```python
from build123d import *

# Parameters (mm, degrees)
SKETCH1_W           = 80
SKETCH1_H           = 65
BOSS_EXTRUDE1_DEPTH = 3
CUT_EXTRUDE1_DEPTH  = 10
CUT_EXTRUDE2_DEPTH  = 10
SKETCH4_R           = 1.5
CUT_EXTRUDE3_DEPTH  = 10
FILLET1_R           = 3
CUT_EXTRUDE4_DEPTH  = 10


with BuildPart() as part:
    # Sketch1 → Boss-Extrude1 (new body)
    with BuildSketch(Plane(origin=(0, 0, 0), x_dir=(1, 0, 0), z_dir=(0, 1, 0))):
        Rectangle(SKETCH1_W, SKETCH1_H)
    extrude(amount=BOSS_EXTRUDE1_DEPTH)

    # Sketch2 → Cut-Extrude1 (cut)
    with BuildSketch(Plane(origin=(0, 0, 0), x_dir=(-1, 0, 0), z_dir=(0, -1, 0))):
        Polygon((22, 32.5), (22, 14.5), (-1, 14.5), (-1, 26.5), (-18, 26.5), (-18, 14.5), (-40, 14.5), (-40, 32.5), align=None)
        Polygon((-1, -26.5), (-18, -26.5), (-18, -14.5), (-40, -14.5), (-40, -32.5), (22, -32.5), (22, -14.5), (-1, -14.5), align=None)
    extrude(amount=-CUT_EXTRUDE1_DEPTH, mode=Mode.SUBTRACT)

    # Sketch3 → Cut-Extrude2 (cut)
    with BuildSketch(Plane(origin=(0, 3, 0), x_dir=(1, 0, 0), z_dir=(0, 1, 0))):
        Polygon((27, -8.3), (9, -8.3), (9, -5.3), (34, -5.3), (34, -10.3), (27, -10.3), align=None)
        Polygon((34, 5.3), (34, 10.3), (27, 10.3), (27, 8.3), (9, 8.3), (9, 5.3), align=None)
    extrude(amount=-CUT_EXTRUDE2_DEPTH, mode=Mode.SUBTRACT)

    # Sketch4 → Cut-Extrude3 (cut)
    with BuildSketch(Plane(origin=(0, 3, 0), x_dir=(1, 0, 0), z_dir=(0, 1, 0))):
        with Locations(Location((-4, 7, 0), (0, 0, 270))):
            Circle(SKETCH4_R)
        with Locations(Location((13.25, 17.9, 0), (0, 0, 270))):
            Circle(SKETCH4_R)
        with Locations(Location((5.75, 17.9, 0), (0, 0, 270))):
            Circle(SKETCH4_R)
        with Locations(Location((37, 7, 0), (0, 0, 270))):
            Circle(SKETCH4_R)
        with Locations(Location((37, 12, 0), (0, 0, 270))):
            Circle(SKETCH4_R)
        with Locations(Location((-19, 12, 0), (0, 0, 270))):
            Circle(SKETCH4_R)
        with Locations(Location((-27.636753237, 17.892684015, 0), (0, 0, 270))):
            Circle(SKETCH4_R)
        with Locations(Location((-34.28355698, 11.245880272, 0), (0, 0, 270))):
            Circle(SKETCH4_R)
        with Locations(Location((-34.28355698, -11.245880272, 0), (0, 0, 270))):
            Circle(SKETCH4_R)
        with Locations(Location((-27.636753237, -17.892684015, 0), (0, 0, 270))):
            Circle(SKETCH4_R)
        with Locations(Location((-19, -12, 0), (0, 0, 270))):
            Circle(SKETCH4_R)
        with Locations(Location((-4, -7, 0), (0, 0, 270))):
            Circle(SKETCH4_R)
        with Locations(Location((5.75, -17.9, 0), (0, 0, 270))):
            Circle(SKETCH4_R)
        with Locations(Location((13.25, -17.9, 0), (0, 0, 270))):
            Circle(SKETCH4_R)
        with Locations(Location((37, -7, 0), (0, 0, 270))):
            Circle(SKETCH4_R)
        with Locations(Location((37, -12, 0), (0, 0, 270))):
            Circle(SKETCH4_R)
    extrude(amount=-CUT_EXTRUDE3_DEPTH, mode=Mode.SUBTRACT)

    # Fillet1
    fillet1_edges = [part.edges().sort_by_distance(p)[0] for p in [
        (-22, 1.5, -14.5),
        (1, 1.5, -14.5),
        (18, 1.5, -14.5),
        (1, 1.5, 14.5),
        (-22, 1.5, 14.5),
        (18, 1.5, 14.5),
    ]]
    fillet(fillet1_edges, radius=FILLET1_R)

    # Sketch5 → Cut-Extrude4 (cut)
    with BuildSketch(Plane(origin=(0, 0, 0), x_dir=(-1, 0, 0), z_dir=(0, -1, 0))):
        Polygon((40, 32.5), (25, 32.5), (40, 17.5), align=None)
        Polygon((40, -17.5), (40, -32.5), (25, -32.5), align=None)
    extrude(amount=-CUT_EXTRUDE4_DEPTH, mode=Mode.SUBTRACT)


solid = part.part
```
Input: part model. Units: mm. Frame: model coordinates. A direction names the side the tool comes from. Give positions to 0.01 mm unless a question says otherwise; leave off trailing zeros. Order: outer loops, then holes, each group sorted by start corner. A loop starts at its lowest first (then second) coordinate and runs counter-clockwise, first axis right, second up. Notation, with made-up numbers: (14, 40) -> (30, 40) arc R29 ccw to (30, 73) -> close; hole circle Ø2 at (-32, 49). An arc over 180 degrees is marked (long way). Write each question's results on one line, items separated by ' | '. Start each with the question number.
Item 1: Contact query for flat-ended pins moving along their axis: P1, Ø2.5, axis at x = 13.25, z = -17.9, coming from the +Y side; P2, Ø1.5, axis at x = 29.5, y = 2, coming from the +Z side; P3, Ø0.9, axis at y = 1, z = -22.5, coming from the -X side. Output: stop coordinate, or through.
Item 2: Cut plane A-A on x = 13.25. Return the cut outline in (y, z), then the cut area to 3 significant figures.
Item 3: Mould query, pull axis X, two halves, no side actions, for faces 1 (the flat face through (40, 1, 0)), 2 (the flat face through (-9, 0, 0)), 3 (the cylindrical face through (0.1, 1.52, -15.36)). Classes: pulls with the +X half, pulls with the -X half, needs draft (parallel to the pull), parting line crosses it, or undercut.
Item 4: Cut plane B-B on z = 7. Return the cut outline in (x, y).
Item 5: Line query: line 1 (X direction, y = 1.15, z = 7); line 2 (Z direction, x = 25, y = 2.05); line 3 (X direction, y = 2.3, z = -25). Output: solid intervals per line, ascending.
Item 6: Set-up query: faces 4 (the cylindrical face through (0.1, 1.52, 15.36)), 5 (the flat face through (18, 1, -22)), 6 (the flat face through (21, 2, 5.3)), 7 (the flat face through (-22, 1, -25)), 8 (the flat face through (30, 1, 14.5)). Return all of +Z, -Z, +X, -X, +Y, -Y with unobstructed straight access to the full face (end or side cutting, diameter ignored); none if empty.
Item 7: Cut plane C-C on x = 30. Return the cut outline in (y, z).
Item 8: Cut plane D-D on z = 24. Return the cut outline in (x, y), then the cut area to 3 significant figures.
Established:
1) P1: through | P2: z = 14.5 | P3: x = -35.45
2) outline: (0, -26.5) -> (3, -26.5) -> (3, -19.4) -> (0, -19.4) -> close; (0, -16.4) -> (3, -16.4) -> (3, -8.3) -> (0, -8.3) -> close; (0, -5.3) -> (3, -5.3) -> (3, 5.3) -> (0, 5.3) -> close; (0, 8.3) -> (3, 8.3) -> (3, 16.4) -> (0, 16.4) -> close; (0, 19.4) -> (3, 19.4) -> (3, 26.5) -> (0, 26.5) -> close | area: 123 mm^2
3) face 1: pulls with the +X half | face 2: needs draft | face 3: undercut
4) outline: (-40, 0) -> (-5.5, 0) -> (-5.5, 3) -> (-40, 3) -> close; (-2.5, 0) -> (9, 0) -> (9, 3) -> (-2.5, 3) -> close; (34, 0) -> (35.5, 0) -> (35.5, 3) -> (34, 3) -> close; (38.5, 0) -> (40, 0) -> (40, 3) -> (38.5, 3) -> close
5) line 1: -40 to -5.5, -2.5 to 9, 34 to 35.5, 38.5 to 40 | line 2: -14.5 to -8.3, -5.3 to 5.3, 8.3 to 14.5 | line 3: -32.5 to -22, 1 to 18
6) face 4: +Z, +Y, -Y | face 5: -Z, +X, +Y, -Y | face 6: +Y, -Y | face 7: -Z, +Y, -Y | face 8: +Z, +X, +Y, -Y
7) outline: (0, -14.5) -> (3, -14.5) -> (3, -10.3) -> (0, -10.3) -> close; (0, -5.3) -> (3, -5.3) -> (3, 5.3) -> (0, 5.3) -> close; (0, 10.3) -> (3, 10.3) -> (3, 14.5) -> (0, 14.5) -> close
8) outline: (-33.5, 0) -> (-22, 0) -> (-22, 3) -> (-33.5, 3) -> close; (1, 0) -> (18, 0) -> (18, 3) -> (1, 3) -> close | area: 85.5 mm^2
